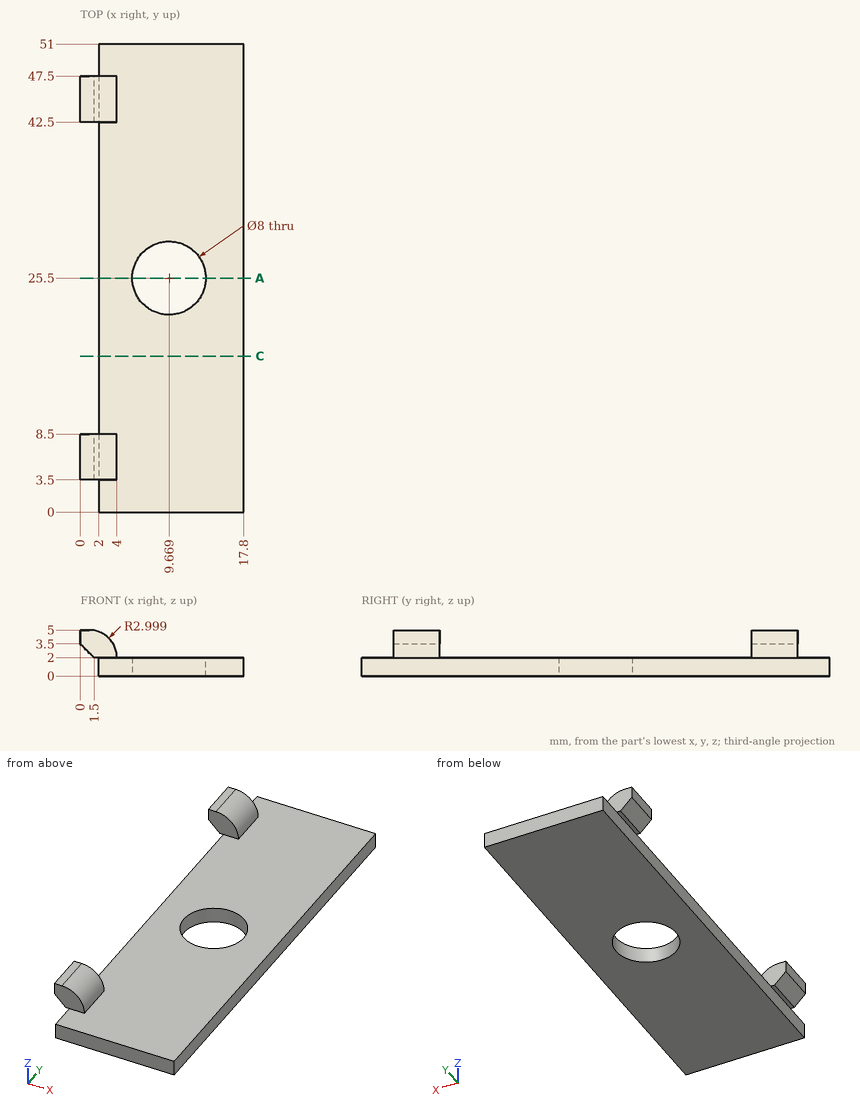
Study the drawing (mm; zero at the part's minimum x, y, z) and answer. Coordinates: 2 decimals unless noted, no trailing zeros. Loops run counter-clockwise (first coordinate to the right, second up) from the corner with the lowest first, then second, coordinate; pieces in that order, holes last. Notation, with made-up numbers: (17.25, 36) -> (66.25, 36) arc R5 ccw to (66.25, 42) -> close; hole circle Ø2 at (33, 89). An arc over 180 degrees is marked (long way). Write item = value, one per line. Start each with the question number.
1) Given P1, Ø0.6, axis at y = 33, z = 1, coming from the -X side; P2, Ø2.5, axis at x = 2.5, z = 4, coming from the -Y side; P3, Ø2.5, axis at x = 1, z = 3, coming from the +Y side, each flat-ended and moving along its own axis, determine where each tip first touches the part or whether it passes through.
2) The part is cut by section C-C, the plane y = 17. Determine the outline of the cut face in (x, z).
3) Find the intervals of material crossed by L1, parallel to X at y = 25.5, z = 0.85; L2, parallel to Z at x = 4.5, y = 20; L3, parallel to Y at x = 2, z = 2.7, in increasing order. Write a range as from..to.
4) The part is cut by section A-A, the plane y = 25.5. Determine the outline of the cut face in (x, z).
Result:
q1.P1 = 2
q1.P2 = 3.5
q1.P3 = 47.5
q2.outline = (2, 0) -> (17.8, 0) -> (17.8, 2) -> (2, 2) -> close
q3.L1 = 2..5.67, 13.67..17.8
q3.L2 = 0..2
q3.L3 = 3.5..8.5, 42.5..47.5
q4.outline = (2, 0) -> (5.67, 0) -> (5.67, 2) -> (2, 2) -> close; (13.67, 0) -> (17.8, 0) -> (17.8, 2) -> (13.67, 2) -> close
